The model under review builds one solid part; all positions refer to its coordinate system, in mm. Face numbers are marked on the shaded views. A direction names the side the tool comes from. Coordinates: 2 decimals unless noted, no trailing zeros. Order: outer loops, then holes, each group sorted by start corner. A loop starts at its lowest first (then second) coordinate and runs counter-clockwise, first axis right, second up. Notation, with made-up numbers: M -29,82.25 L -12,82.25 A19 cw -12,94.25 Z; hole C 68,9 d10. An arc over 180 degrees is marked long. Answer as CSV lines item,"result". Start each with the question number.
Q1. The part is to be moulded in two halves that separate along X. For the marked faces 1, 2 and 3, say which applies: +X half, -X half, draft (parallel to the pull), parting line (faces both ways), or undercut.
Q2. Consider section B-B on z = 33.5. Write out the cut boundary in (x, y).
Q3. Machinability: for the marked faces 4 and 5, which of the approach directions +Z, -Z, +X, -X, +Y, -Y give a long, thin tool a straight path to every point of the face, cutting with its end or side? Answer none if there is none.
Q4. Consider section C-C on z = 57. Write out the cut boundary in (x, y).
Q5. Wall thickness on L1, parallel to X at y = 23.5, z = 42.5; L2, parallel to Z at x = -36, y = 26; L3, parallel to X at y = 39, z = 48: over which ranges is each line inside the solid? List them lowest first. Write a range as [from, to].
Q6. Consider section D-D on y = 10. Write out the cut boundary in (x, z), and give its area (3 significant figures).
Q7. For P1, Ø12, axis at y = 27.5, z = 25, coming from the -X side; P2, Ø4, axis at y = 13.5, z = 29.5, coming from the -X side; P3, Ø6, axis at y = 39.5, z = 26, coming from the -X side, all flat-tipped, find the tip position at first contact; note any pin that passes through.
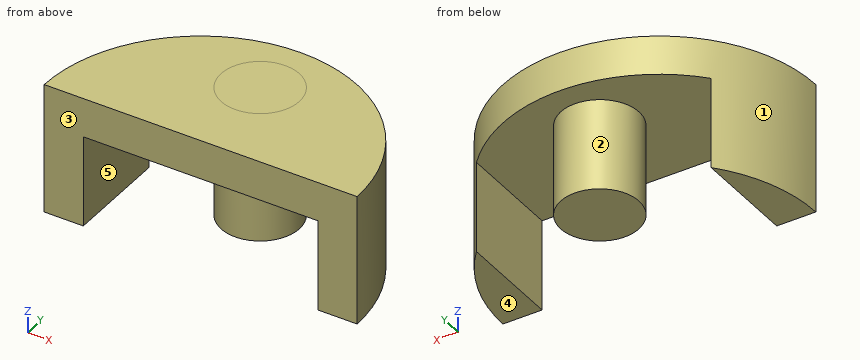
from build123d import *

# Parameters (mm, degrees)
BOSS_EXTRUDE1_DEPTH = 65
CUT_EXTRUDE1_START  = -60
SKETCH4_W           = 90
SKETCH4_H           = 35
CUT_EXTRUDE1_DEPTH  = 60
BOSS_EXTRUDE2_START = -50
SKETCH5_R           = 15
BOSS_EXTRUDE2_DEPTH = 50.000012
SKETCH7_W           = 120
SKETCH7_H           = 15
CUT_EXTRUDE3_DEPTH  = 61


with BuildPart() as part:
    # Sketch3 → Boss-Extrude1 (new body)
    with BuildSketch(Plane.XY):
        with BuildLine():
            Line((-60, 0), (60, 0))
            ThreePointArc((60, 0), (0, 60), (-60, 0))
        make_face()
    extrude(amount=BOSS_EXTRUDE1_DEPTH)

    # Sketch4 → Cut-Extrude1 (cut)
    with BuildSketch(Plane.XZ.offset(CUT_EXTRUDE1_START)):
        with Locations((0, 32.5)):
            Rectangle(SKETCH4_W, SKETCH4_H)
    extrude(amount=CUT_EXTRUDE1_DEPTH, mode=Mode.SUBTRACT)

    # Sketch5 → Boss-Extrude2 (add)
    with BuildSketch(Plane.XY.offset(65).offset(BOSS_EXTRUDE2_START)):
        with Locations((0, 36.035216542)):
            Circle(SKETCH5_R)
    extrude(amount=BOSS_EXTRUDE2_DEPTH)

    # Sketch7 → Cut-Extrude3 (cut, through all)
    with BuildSketch(Plane.XZ):
        with Locations((0, 7.5)):
            Rectangle(SKETCH7_W, SKETCH7_H)
    extrude(amount=-CUT_EXTRUDE3_DEPTH, mode=Mode.SUBTRACT)


solid = part.part
Evaluation:
1,face 1,"parting line"
1,face 2,"undercut"
1,face 3,"draft"
2,outline,"M -60,0 L -45,0 L -45,39.69 A60 ccw Z; C 0,36.04 d30; M 45,0 L 60,0 A60 ccw 45,39.69 Z"
3,face 4,"-Z, +X, -X, +Y, -Y"
3,face 5,"-Z, +Y, -Y"
4,outline,"M -60,0 L 60,0 A60 ccw Z"
5,L1,"x = [-55.21, -45], [-8.24, 8.24], [45, 55.21]"
5,L2,"z = [50, 65]"
5,L3,"x = [-45.6, -45], [-14.7, 14.7], [45, 45.6]"
6,outline,"M -59.16,15 L -45,15 L -45,50 L 45,50 L 45,15 L 59.16,15 L 59.16,65 L -59.16,65 Z"
6,area,"2,770 mm²"
7,P1,"stops at x = -56.02"
7,P2,"stops at x = -58.89"
7,P3,"stops at x = -47.62"
